Verification items for the finished model (mm, model axes). Face numbers are marked on the shaded views. A direction names the side the tool comes from. Coordinates: 2 decimals unless noted, no trailing zeros. Order: outer loops, then holes, each group sorted by start corner. A loop starts at its lowest first (then second) coordinate and runs counter-clockwise, first axis right, second up. Notation, with made-up numbers: M 78,-15.75 L 85,-15.75 A28 cw 85,8.25 Z; hole C 4,-19 d1. An arc over 180 degrees is marked long. Return JSON: item names as keys, results as strings. Group by question number.
1. Section check B-B, the plane z = 20. Record the cut outline in (x, y).
2. Section check C-C, the plane x = -24.25. Record the cut outline in (y, z), plus the area to 3 significant figures.
3. Material ranges on line 1 along Y through (x, z) = (-30.25, 24); line 2 along X through (y, z) = (43.5, 40.5); line 3 along Y through (x, z) = (-21.25, 6.5), recorded low to high.
4. Section check D-D, the plane z = 13. Record the cut outline in (x, y), plus the area to 3 significant figures.
5. Gauge pin test, flat end, axial feed: pin 1 (13.5 mm diameter, centred on y = -6, z = 25, fed in from +X). Record the tip position at first contact, or that the pin passes through.
6. Section check A-A, the plane y = 37.5. Record the cut outline in (x, z).
7. Mould release check, pull along Y, two halves, no side actions. Record for the marked faces 4, 5 and 6: +Y half, -Y half, draft (parallel to the pull), parting line (faces both ways), or undercut.
8. Set-up check for the marked faces 1, 2 and 3: record each of +Z, -Z, +X, -X, +Y, -Y from which the full face is reachable in a straight line by a thin tool's end or side.
```python
from build123d import *

# Parameters (mm, degrees)
SKETCH1_W           = 100
SKETCH1_H           = 75
BOSS_EXTRUDE1_DEPTH = 45
SKETCH2_W           = 15
SKETCH2_H           = 25
CUT_EXTRUDE1_DEPTH  = 78.014609004
SKETCH3_W           = 30.197143083
SKETCH3_H           = 100
CUT_EXTRUDE2_DEPTH  = 78.014609004
SKETCH4_W           = 17
SKETCH4_H           = 32
CUT_EXTRUDE3_DEPTH  = 16


with BuildPart() as part:
    # Sketch1 → Boss-Extrude1 (new body)
    with BuildSketch(Plane(origin=(0, 0, 0), x_dir=(0, 1, 0), z_dir=(0, 0, 1))):
        Rectangle(SKETCH1_W, SKETCH1_H)
    extrude(amount=BOSS_EXTRUDE1_DEPTH)

    # Sketch2 → Cut-Extrude1 (cut, through all)
    with BuildSketch(Plane.XY.offset(45)):
        Polygon((-15.5, 18), (-32.5, 18), (-32.5, -45), (32.5, -45), (32.5, 45), (-15.5, 45), (-15.5, 20), align=None)
        with Locations((-25, 32.5)):
            Rectangle(SKETCH2_W, SKETCH2_H)
    extrude(amount=-CUT_EXTRUDE1_DEPTH, mode=Mode.SUBTRACT)

    # Sketch3 → Cut-Extrude2 (cut, through all)
    with BuildSketch(Plane.XY.offset(45)):
        with Locations((-0.401428459, 0)):
            Rectangle(SKETCH3_W, SKETCH3_H)
    extrude(amount=-CUT_EXTRUDE2_DEPTH, mode=Mode.SUBTRACT)


with BuildPart() as cut_extrude2_kept_piece:
    # of the separate pieces the step leaves, the one the design keeps (cut_extrude2_pieces_kept)
    add(part.part.solids().sort_by_distance((-37.5, -50, 0))[0])

    # Sketch4 → Cut-Extrude3 (cut)
    with BuildSketch(Plane.XY):
        with Locations((-24, 34)):
            Rectangle(SKETCH4_W, SKETCH4_H)
    extrude(amount=CUT_EXTRUDE3_DEPTH, mode=Mode.SUBTRACT)


solid = cut_extrude2_kept_piece.part
```
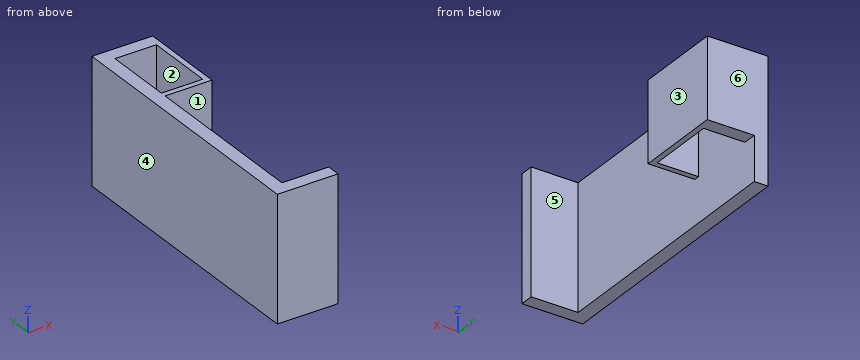
Answers follow:
{
 "1": {"outline": "M -37.5,-50 L -15.5,-50 L -15.5,-45 L -32.5,-45 L -32.5,18 L -15.5,18 L -15.5,50 L -37.5,50 Z; hole M -32.5,20 L -17.5,20 L -17.5,45 L -32.5,45 Z"},
 "2": {"outline": "M -50,0 L -45,0 L -45,45 L -50,45 Z; M 18,16 L 20,16 L 20,45 L 18,45 Z; M 45,16 L 50,16 L 50,45 L 45,45 Z", "area": "428 mm^2"},
 "3": {"line 1": "-50 to -45, 18 to 20, 45 to 50", "line 2": "-37.5 to -32.5, -17.5 to -15.5", "line 3": "-50 to -45"},
 "4": {"outline": "M -37.5,-50 L -15.5,-50 L -15.5,-45 L -32.5,-45 L -32.5,50 L -37.5,50 Z", "area": "585 mm^2"},
 "5": {"pin 1": "x = -32.5"},
 "6": {"outline": "M -37.5,0 L -32.5,0 L -32.5,45 L -37.5,45 Z; M -17.5,16 L -15.5,16 L -15.5,45 L -17.5,45 Z"},
 "7": {"face 4": "draft", "face 5": "undercut", "face 6": "+Y half"},
 "8": {"face 1": "+Z, -Z, +X", "face 2": "+Z, -Z", "face 3": "+Z, -Z, +X, +Y, -Y"}
}
